from build123d import *

# Parameters (mm, degrees)
SKETCH_W     = 1226
SKETCH_H     = 690
PAD_DEPTH    = 60
SKETCH001_W  = 1178.222099
SKETCH001_H  = 634.606854
POCKET_DEPTH = 5


with BuildPart() as part:
    # Sketch → Pad (new body)
    with BuildSketch(Plane.YZ):
        with Locations((613, 345)):
            Rectangle(SKETCH_W, SKETCH_H)
    extrude(amount=PAD_DEPTH)

    # Sketch001 (on Face6 of Pad) → Pocket (cut)
    with BuildSketch(Plane.YZ.offset(60)):
        with Locations((610.844516, 346.005472)):
            Rectangle(SKETCH001_W, SKETCH001_H)
    extrude(amount=-POCKET_DEPTH, mode=Mode.SUBTRACT)


solid = part.part
Input: part model. Units: mm. Frame: model coordinates. Round coordinates to 2 decimals unless told otherwise and drop trailing zeros. Loops run counter-clockwise (first coordinate to the right, second up) from the corner with the lowest first, then second, coordinate; pieces in that order, holes last. Notation, with made-up numbers: M -28.75,13 L -20.75,13 A27 cw -20.75,30 Z; hole C -15.5,-33.75 d7. An arc over 180 degrees is marked long. Answer as CSV lines item,"result". Start each with the question number.
(1) Section B-B, the plane y = 847.5. Output: boundary loops of the cut face in (x, z).
(2) First-contact query: pin 1 (3 mm diameter, centred on y = 786.5, z = 441, fed in from +X). Flat tip, straight axial feed; report the tip coordinate or a pass-through.
(3) Draft query along Z for faces 1 (the flat face through (55, 603, 350)), 2 (the flat face through (60, 565, 14)), 3 (the flat face through (30, 604, 690)). Return one class per face: released by +Z, released by -Z, zero draft, split by the parting line, or undercut.
(4) Section A-A, the plane z = 609. Output: boundary loops of the cut face in (x, y).
(5) Line query: line 1 (X direction, y = 486, z = 428.5). Output: solid intervals per line, ascending. Write a range as [from, to].
Values found:
1,outline,"M 0,0 L 60,0 L 60,28.7 L 55,28.7 L 55,663.31 L 60,663.31 L 60,690 L 0,690 Z"
2,pin 1,"stops at x = 55"
3,face 1,"undercut"
3,face 2,"zero draft"
3,face 3,"released by +Z"
4,outline,"M 0,0 L 60,0 L 60,21.73 L 55,21.73 L 55,1199.96 L 60,1199.96 L 60,1226 L 0,1226 Z"
5,line 1,"x = [0, 55]"
